Geometry: final body of the model. Coordinates: model frame, mm. A direction names the side the tool comes from. Give positions to 0.01 mm unless a question says otherwise; leave off trailing zeros. Write each loop counter-clockwise with the first axis right and the second up, starting at its lowest first coordinate (ties: lowest second). Pieces come first, ordered by that corner, then holes.
Q1. Mould query, pull axis X, two halves, no side actions, for faces 1 (the cylindrical face through (2.38, 10.74, -1.48)), 2 (the cylindrical face through (10.316, 7.91, 0.042)), 3 (the flat face through (-3, 0, 3)). Classes: +X half, -X half, draft (parallel to the pull), parting line (faces both ways), or undercut.
Q2. Line query: line 1 (Y direction, x = 0, z = 1.55); line 2 (Y direction, x = 0, z = -1.5); line 3 (Z direction, x = -10, y = 2.25). Output: solid intervals per line, ascending.
Q3. Section D-D (y = -10). Return the cut outline in (x, z), plus the area to 3 significant figures.
Q4. Reachability of faces 4 (the cylindrical face through (-0.54, -2.44, 1.52)), 5 (the flat face through (0, 3, 0)) from +Z, -Z, +X, -X, +Y, -Y: full face, straight path, thin tool, end or side. Return the list, or none.
Q5. Pin query (flat end, axial travel): pin 1 Ø3 at (x, z) = (-2, 1) entering from +Y; pin 2 Ø1 at (x, z) = (-9, -2) entering from +Y. Return the tip coordinate at first contact, or that it passes through.
Q6. Section C-C (z = -1). Return the cut outline in (x, y).
Q7. Section A-A (x = 0). Return the cut outline in (y, z).
Autodesk Inventor part; units mm, degrees
ref_plane "YZ Plane" through (0, 0, 0) normal (1, 0, 0) x (0, 1, 0)
ref_plane "XZ Plane" through (0, 0, 0) normal (0, 1, 0) x (-1, 0, 0)
ref_plane "XY Plane" through (0, 0, 0) normal (0, 0, 1) x (1, 0, 0)
sketch "Sketch1" plane through (0, 0, 0) normal (0, 0, 1) x (1, 0, 0)
  circle A0 centre (0, 0) radius 10.75
  point P0 (0, 0)
extrude "Extrusion1" add sketch "Sketch1" along normal blind 3
sketch "Sketch2" plane through (0, 0, 3) normal (0, 0, 1) x (1, 0, 0)
  circle A0 centre (0, 0) radius 10.75
  circle A1 centre (0, 0) radius 2.5
  dimension "d2" = 5
extrude "Extrusion2" cut sketch "Sketch2" against normal blind 3 contours A1
sketch "Sketch3" plane through (0, 0, 0) normal (0, 0, -1) x (-1, 0, 0)
  circle A0 centre (0, 0) radius 10.75
  circle A1 centre (0, 0) radius 13
  dimension "d5" = 26
extrude "Extrusion3" add sketch "Sketch3" against normal up to surface (3 mm away)
sketch "Sketch4" plane through (0, 0, 0) normal (0, 0, -1) x (-1, 0, 0)
  circle A0 centre (0, 0) radius 13
  circle A1 centre (0, 0) radius 2.5
  circle A2 centre (0, 0) radius 11
  dimension "d8" = 22
extrude "Extrusion4" add sketch "Sketch4" along normal blind 3 contours A0
properties part number "HubCover"
Computed:
1. face 1: undercut
1. face 2: parting line
1. face 3: draft
2. line 1: y = -13 to -2.5, 2.5 to 13
2. line 2: y = -13 to -11, 11 to 13
2. line 3: z = 0 to 3
3. outline: (-8.31, -3) - (-4.58, -3) - (-4.58, 0) - (4.58, 0) - (4.58, -3) - (8.31, -3) - (8.31, 3) - (-8.31, 3) - close
3. area: 72.2 mm2
4. face 4: +Z, -Z
4. face 5: -Z
5. pin 1: stops at y = 12.99
5. pin 2: stops at y = 9.84
6. outline: circle Ø26 at (0, 0); hole circle Ø22 at (0, 0)
7. outline: (-13, -3) - (-11, -3) - (-11, 0) - (-2.5, 0) - (-2.5, 3) - (-13, 3) - close; (2.5, 0) - (11, 0) - (11, -3) - (13, -3) - (13, 3) - (2.5, 3) - close
